The model under review builds one solid part; all positions refer to its coordinate system, in mm. A direction names the side the tool comes from. Give positions to 0.01 mm unless a question says otherwise; leave off trailing zeros. Loops run counter-clockwise (first coordinate to the right, second up) from the corner with the lowest first, then second, coordinate; pieces in that order, holes last. Notation, with made-up numbers: M 38.25,74 L 75.25,74 A36 cw 75.25,112 Z; hole C 45.5,20.5 d7. An arc over 180 degrees is marked long. Put each result on its own line as item: value. Start each with the question number.
```python
from build123d import *

# Parameters (mm, degrees)
SKETCH_1_W          = 60
SKETCH_1_H          = 30
EXTRUDE_1_DEPTH     = 7
CUT_EXTRUDE_1_REACH = 69.446
SKETCH_2_R          = 5
SKETCH_3_W          = 7
SKETCH_3_H          = 18
EXTRUDE_2_DEPTH     = 18
SKETCH_4_W          = 7
SKETCH_4_H          = 18
EXTRUDE_3_DEPTH     = 18
CUT_EXTRUDE_2_REACH = 73.589
SKETCH_5_R          = 3
FILLET_2_SIZE       = 20
FILLET_2_SIZE_2     = 5
FILLET_3_DEPTH      = 27.0000001
FILLET_START        = -1
FILLET_3_2_DEPTH    = 32
FILLET_4_R          = 5
FILLET_5_R          = 5
FILLET_6_R          = 5
FILLET_7_R          = 5
FILLET_8_R          = 10


with BuildPart() as part:
    # 草图1 → 凸台-拉伸1 (new body)
    with BuildSketch(Plane.XY):
        with Locations((30, 15)):
            Rectangle(SKETCH_1_W, SKETCH_1_H)
    extrude(amount=EXTRUDE_1_DEPTH)

    # 草图2 → 切除-拉伸1 (cut, up to next)
    with BuildSketch(Plane(origin=(0, 0, 0), x_dir=(-1, 0, 0), z_dir=(0, 0, -1)), mode=Mode.PRIVATE) as cut_extrude_1_sk1:
        with Locations((-50, 15)):
            Circle(SKETCH_2_R)
    cut_extrude_1_tool1 = extrude(cut_extrude_1_sk1.sketch, amount=-CUT_EXTRUDE_1_REACH, mode=Mode.PRIVATE) & part.part
    add(cut_extrude_1_tool1.solids().sort_by_distance((50, 15, 0))[0], mode=Mode.SUBTRACT)

    # 草图3 → 凸台-拉伸2 (add)
    with BuildSketch(Plane.XY.offset(7)):
        with Locations((3.5, 15)):
            Rectangle(SKETCH_3_W, SKETCH_3_H)
    extrude(amount=EXTRUDE_2_DEPTH)

    # 草图4 → 凸台-拉伸3 (add)
    with BuildSketch(Plane(origin=(0, 0, 0), x_dir=(-1, 0, 0), z_dir=(0, 0, -1))):
        with Locations((-3.5, 15)):
            Rectangle(SKETCH_4_W, SKETCH_4_H)
    extrude(amount=EXTRUDE_3_DEPTH)

    # 草图5 → 切除-拉伸2 (cut, up to next)
    with BuildSketch(Plane.ZY, mode=Mode.PRIVATE) as cut_extrude_2_sk1:
        with Locations((-11, 15)):
            Circle(SKETCH_5_R)
    cut_extrude_2_tool1 = extrude(cut_extrude_2_sk1.sketch, amount=-CUT_EXTRUDE_2_REACH, mode=Mode.PRIVATE) & part.part
    # 草图5 → 切除-拉伸2 (cut, up to next)
    with BuildSketch(Plane.ZY, mode=Mode.PRIVATE) as cut_extrude_2_sk2:
        with Locations((18, 15)):
            Circle(SKETCH_5_R)
    cut_extrude_2_tool2 = extrude(cut_extrude_2_sk2.sketch, amount=-CUT_EXTRUDE_2_REACH, mode=Mode.PRIVATE) & part.part
    add(cut_extrude_2_tool1.solids().sort_by_distance((0, 15, -11))[0], mode=Mode.SUBTRACT)
    add(cut_extrude_2_tool2.solids().sort_by_distance((0, 15, 18))[0], mode=Mode.SUBTRACT)

    # 圆角2
    # a fillet whose section is not a circle: 20, 5 mm, written as the material it adds along each edge
    with BuildSketch(Plane(origin=(7, 24, 7), x_dir=(1, 0, 0), z_dir=(0, -1, 0))) as fillet_2_piece_1:
        with BuildLine():
            Bezier((FILLET_2_SIZE, 0), (0, 0), (0, FILLET_2_SIZE_2), weights=[1, 0.707106781, 1])
            Line((0, FILLET_2_SIZE_2), (0, 0))
            Line((0, 0), (FILLET_2_SIZE, 0))
        make_face()
    extrude(amount=18)
    with BuildSketch(Plane(origin=(7, 24, 0), x_dir=(1, 0, 0), z_dir=(0, -1, 0))) as fillet_2_piece_2:
        with BuildLine():
            Bezier((FILLET_2_SIZE, 0), (0, 0), (0, -FILLET_2_SIZE_2), weights=[1, 0.707106781, 1])
            Line((0, -FILLET_2_SIZE_2), (0, 0))
            Line((0, 0), (FILLET_2_SIZE, 0))
        make_face()
    extrude(amount=18)

    # 圆角3: read off the stored shape, not the designer's step
    # 圆角3 outline → 圆角3 (add)
    with BuildSketch(Plane.YZ):
        with BuildLine():
            Line((24, 25), (24, 7))
            Line((24, 7), (30, 7))
            ThreePointArc((30, 7), (25.539501058, 15.513167019), (24, 25))
        make_face()
        with BuildLine():
            ThreePointArc((6, 25), (4.460498942, 15.513167019), (0, 7))
            Line((0, 7), (6, 7))
            Line((6, 7), (6, 25))
        make_face()
        with BuildLine():
            Line((24, 0), (24, -18))
            ThreePointArc((24, -18), (25.539501058, -8.513167019), (30, 0))
            Line((30, 0), (24, 0))
        make_face()
        with BuildLine():
            Line((6, -18), (6, 0))
            Line((6, 0), (0, 0))
            ThreePointArc((0, 0), (4.460498942, -8.513167019), (6, -18))
        make_face()
    extrude(amount=FILLET_3_DEPTH)

    # Fillet 3 2 outline → Fillet 3 2 (cut)
    with BuildSketch(Plane(origin=(0, 0, 0), x_dir=(1, 0, 0), z_dir=(0, 1, 0)).offset(FILLET_START)):
        with BuildLine():
            add(Edge.make_bspline(
                [(7, -12), (7, -7), (27, -7)],
                knots=[0, 0, 0, 1, 1, 1], degree=2, weights=[1, 0.707106781, 1]))
            Line((7, -12), (7, -25))
            Line((7, -25), (27.0000001, -25))
            Line((27.0000001, -25), (27, -7))
        make_face()
        with BuildLine():
            Line((27.0000001, 18), (7, 18))
            Line((7, 18), (7, 5))
            add(Edge.make_bspline(
                [(27, 0), (7, 0), (7, 5)],
                knots=[0, 0, 0, 1, 1, 1], degree=2, weights=[1, 0.707106781, 1]))
            Line((27, 0), (27.0000001, 18))
        make_face()
    extrude(amount=FILLET_3_2_DEPTH, mode=Mode.SUBTRACT)

    # 圆角4
    fillet_4_edges = [part.edges().sort_by_distance(p)[0] for p in [
        (3.5, 24, 25),
    ]]
    fillet(fillet_4_edges, radius=FILLET_4_R)

    # 圆角5
    fillet_5_edges = [part.edges().sort_by_distance(p)[0] for p in [
        (3.5, 6, 25),
    ]]
    fillet(fillet_5_edges, radius=FILLET_5_R)

    # 圆角6
    fillet_6_edges = [part.edges().sort_by_distance(p)[0] for p in [
        (3.5, 6, -18),
    ]]
    fillet(fillet_6_edges, radius=FILLET_6_R)

    # 圆角7
    fillet_7_edges = [part.edges().sort_by_distance(p)[0] for p in [
        (3.5, 24, -18),
    ]]
    fillet(fillet_7_edges, radius=FILLET_7_R)

    # 圆角8
    fillet_8_edges = [part.edges().sort_by_distance(p)[0] for p in [
        (60, 0, 3.5),
        (60, 30, 3.5),
    ]]
    fillet(fillet_8_edges, radius=FILLET_8_R)


solid = part.part
```
Item 1: Consider section A-A, the plane z = -9.5. Write out the cut boundary in (x, y), plus the area to 3 significant figures.
Item 2: Draft analysis for pull direction Y (two halves, no side actions). For faces 1 (the cylindrical face through (54, 12, 3)), 2 (the flat face through (4, 15, -18)), 3 (the cylindrical face through (56.99, 27.15, 3.55)), state which applies: +Y half, -Y half, draft (parallel to the pull), parting line (faces both ways), or undercut.
Item 3: Clearance check with flat-ended pins moving along their axes: pin 1 Ø6 at (x, y) = (51.5, 26.5) entering from -Z; pin 2 Ø1 at (y, z) = (27, 13) entering from -X; pin 3 Ø15 at (x, y) = (51.5, 19) entering from +Z; pin 4 Ø6.5 at (y, z) = (11.5, 18) entering from +X. State where each tip first meets the part, or that it passes through.
Item 4: Tool access review of faces 4 (the cylindrical face through (5.44, 3.25, -5.45)), 5 (the flat face through (7, 12, 17)), 6 (the flat face through (7, 17.5, -13)): name each direction out of +Z, -Z, +X, -X, +Y, -Y from which nothing blocks a thin tool from reaching the whole face with its end or side.
Item 5: Consider section C-C, the plane y = 15. Give the number of separate pieces and of enclosed holes in the cut face, plus the area to 3 significant figures.
Item 6: Consider section D-D, the plane x = 41.5. Write out the cut boundary in (y, z), plus the area to 3 significant figures.
Item 7: To check wall thickness, follow L1, parallel to Z at x = 40.5, y = 12; L2, parallel to Y at x = 4, z = 18. State the ranges of each line that lie inside material, in increasing order. Write a range as [from, to].
Item 8: Consider section B-B, the plane z = 4.5. Write out the cut boundary in (x, y), plus the area to 3 significant figures.
Report:
1. outline: M 0,4.77 L 7,4.77 L 7,12.4 L 0,12.4 Z; M 0,17.6 L 7,17.6 L 7,25.23 L 0,25.23 Z
1. area: 107 mm²
2. face 1: undercut
2. face 2: draft
2. face 3: +Y half
3. pin 1: z = 0
3. pin 2: x = 0
3. pin 3: z = 7
3. pin 4: x = 7
4. face 4: -Z, +X, -X, -Y
4. face 5: +Z, +X, +Y, -Y
4. face 6: -Z, +X, +Y, -Y
5. separate pieces: 4
5. enclosed holes: 0
5. area: 561 mm²
6. outline: M 0,0 L 30,0 L 30,7 L 0,7 Z
6. area: 210 mm²
7. L1: [0, 7]
7. L2: [5.17, 12], [18, 24.83]
8. outline: M 0,0 L 50,0 A10 ccw 60,10 L 60,20 A10 ccw 50,30 L 0,30 Z; hole C 50,15 d10
8. area: 1,680 mm²
